```python
from build123d import *

# Parameters (mm, degrees)
BOSS_EXTRUDE3_DEPTH      = 18
BOSS_EXTRUDE3_DEPTH_BACK = 18
SKETCH1_R                = 5
BOSS_EXTRUDE4_DEPTH      = 3
BOSS_EXTRUDE4_DEPTH_BACK = 3
SKETCH1_5_R              = 5
SKETCH1_5_R_2            = 3
SKETCH3_W                = 40.653147646
SKETCH3_H                = 22
CUT_EXTRUDE2_DEPTH       = 48.581509013


with BuildPart() as part:
    # Sketch1 → Boss-Extrude3 (new, two sides: drawn at the far end of the back side and taken through both)
    with BuildSketch(Plane(origin=(0, 0, 0), x_dir=(1, 0, 0), z_dir=(0, 1, 0)).offset(-BOSS_EXTRUDE3_DEPTH_BACK)):
        with BuildLine():
            Line((0, 10), (0, -10))
            Line((0, -10), (0, -14))
            Line((0, -14), (8, -14))
            Line((8, -14), (26.271311561, -9.738641784))
            ThreePointArc((26.271311561, -9.738641784), (34, 0), (26.271311561, 9.738641784))
            Line((26.271311561, 9.738641784), (8, 14))
            Line((8, 14), (0, 14))
            Line((0, 14), (0, 10))
        make_face()
        with Locations(Location((24, 0, 0), (0, 0, 270))):
            Circle(SKETCH1_R, mode=Mode.SUBTRACT)
    extrude(amount=BOSS_EXTRUDE3_DEPTH + BOSS_EXTRUDE3_DEPTH_BACK)

    # Sketch1_5 → Boss-Extrude4 (add, two sides: drawn at the far end of the back side and taken through both)
    # profile 1 of 2: a face of its own
    with BuildSketch(Plane(origin=(0, 0, 0), x_dir=(1, 0, 0), z_dir=(0, 1, 0)).offset(-BOSS_EXTRUDE4_DEPTH_BACK)):
        Polygon((-30, 6.5), (-30, -6.5), (-20, -10), (0, -10), (0, 10), (-20, 10), align=None)
        with Locations(Location((-20, 0, 0), (0, 0, 270))):
            Circle(SKETCH1_5_R, mode=Mode.SUBTRACT)
        with Locations(Location((-7, 0, 0), (0, 0, 270))):
            Circle(SKETCH1_5_R_2, mode=Mode.SUBTRACT)
    # profile 2 of 2: a face of its own
    with BuildSketch(Plane(origin=(0, 0, 0), x_dir=(1, 0, 0), z_dir=(0, 1, 0)).offset(-BOSS_EXTRUDE4_DEPTH_BACK)):
        with BuildLine():
            Line((0, 10), (0, -10))
            Line((0, -10), (0, -14))
            Line((0, -14), (8, -14))
            Line((8, -14), (26.271311561, -9.738641784))
            ThreePointArc((26.271311561, -9.738641784), (34, 0), (26.271311561, 9.738641784))
            Line((26.271311561, 9.738641784), (8, 14))
            Line((8, 14), (0, 14))
            Line((0, 14), (0, 10))
        make_face()
        with Locations(Location((24, 0, 0), (0, 0, 270))):
            Circle(SKETCH1_5_R, mode=Mode.SUBTRACT)
    extrude(amount=BOSS_EXTRUDE4_DEPTH + BOSS_EXTRUDE4_DEPTH_BACK)

    # Sketch3 → Cut-Extrude2 (cut, through all)
    with BuildSketch(Plane(origin=(0, 0, -14), x_dir=(-1, 0, 0), z_dir=(0, 0, -1))):
        with Locations((-28.326573823, 0)):
            Rectangle(SKETCH3_W, SKETCH3_H)
    extrude(amount=-CUT_EXTRUDE2_DEPTH, mode=Mode.SUBTRACT)


solid = part.part
```
Input: part model. Units: mm. Frame: model coordinates. A direction names the side the tool comes from. Round coordinates to 2 decimals unless told otherwise and drop trailing zeros. Loops run counter-clockwise (first coordinate to the right, second up) from the corner with the lowest first, then second, coordinate; pieces in that order, holes last. Notation, with made-up numbers: (28.25, 21.25) -> (48.25, 21.25) arc R10 ccw to (48.25, 32.25) -> close; hole circle Ø2 at (57, 20). An arc over 180 degrees is marked (long way). Use one line per item in the form item = value. Start each with the question number.
Item 1: Material intervals for L1, parallel to Y at x = 19, z = 3.25; L2, parallel to X at y = -13.75, z = 0; L3, parallel to Z at x = -16, y = 0, sorted ascending. Write a range as from..to.
Item 2: Section query C-C on y = -16. Return the cut outline in (x, z).
Item 3: Section query B-B on z = 0. Return the cut outline in (x, y).
Item 4: Contact query for flat-ended pins moving along their axis: pin 1 Ø11.5 at (x, z) = (-20, 0) entering from +Y; pin 2 Ø1 at (y, z) = (12.5, 5) entering from -X; pin 3 Ø1.8 at (x, y) = (-11, 0) entering from -Z; pin 4 Ø8 at (x, z) = (24, 0) entering from -Y. Output: stop coordinate, or through.
Item 5: Section query D-D on y = 0. Return the cut outline in (x, z).
Item 6: Set-up query: faces 4 (the face through (17.26, -14.55, -11.84)), 5 (the face through (18, 11, 0)), 6 (the face through (-10, 0, 10)), 7 (the face through (-24.88, -0.04, -1.08)), 8 (the face through (-15, 3, 2)). Return all of +Z, -Z, +X, -X, +Y, -Y with unobstructed straight access to the full face (end or side cutting, diameter ignored); none if empty.
Item 7: Mould query, pull axis X, two halves, no side actions, for faces 1 (the face through (19.12, -14.55, -1.08)), 2 (the face through (-10, 0, -10)), 3 (the face through (8, 0, 0)). Classes: pulls with the +X half, pulls with the -X half, needs draft (parallel to the pull), parting line crosses it, or undercut.
Item 8: Section query A-A on x = -7. Return the cut outline in (y, z), then the cut area to 3 significant figures.
Ans:
q1.L1 = -18..-11, 11..18
q1.L2 = 0..19, 29..34
q1.L3 = -10..-3, 3..10
q2.outline = (0, -14) -> (8, -14) -> (26.27, -9.74) arc R10 ccw to (26.27, 9.74) -> (8, 14) -> (0, 14) -> close; hole circle Ø10 at (24, 0)
q3.outline = (-30, -3) -> (-25, -3) -> (-25, 3) -> (-30, 3) -> close; (-15, -3) -> (-10, -3) -> (-10, 3) -> (-15, 3) -> close; (-4, -3) -> (0, -3) -> (0, -18) -> (19, -18) -> (19, -11) -> (8, -11) -> (8, 11) -> (19, 11) -> (19, 18) -> (0, 18) -> (0, 3) -> (-4, 3) -> close; (29, -18) -> (34, -18) -> (34, -11) -> (29, -11) -> close; (29, 11) -> (34, 11) -> (34, 18) -> (29, 18) -> close
q4.pin_1 = 3
q4.pin_2 = 0
q4.pin_3 = -10
q4.pin_4 = through
q5.outline = (-30, -6.5) -> (-20, -10) -> (0, -10) -> (0, -14) -> (8, -14) -> (8, 14) -> (0, 14) -> (0, 10) -> (-20, 10) -> (-30, 6.5) -> close; hole circle Ø10 at (-20, 0); hole circle Ø6 at (-7, 0)
q6.face_4 = -Z, +X, +Y, -Y
q6.face_5 = +Z, -Z, +X
q6.face_6 = +Z, -X, +Y, -Y
q6.face_7 = +Y, -Y
q6.face_8 = +Z, -Z, -X, +Y
q7.face_1 = undercut
q7.face_2 = needs draft
q7.face_3 = pulls with the +X half
q8.outline = (-3, -10) -> (3, -10) -> (3, -3) -> (-3, -3) -> close; (-3, 3) -> (3, 3) -> (3, 10) -> (-3, 10) -> close
q8.area = 84.0 mm^2
